Part model, mm, in its own coordinate system. Face numbers are marked on the shaded views. A direction names the side the tool comes from. Round coordinates to 2 decimals unless told otherwise and drop trailing zeros. Write each loop counter-clockwise with the first axis right and the second up, starting at its lowest first coordinate (ties: lowest second). Pieces come first, ordered by that corner, then holes. Notation, with made-up numbers: M 86.5,-4.75 L 118.5,-4.75 A17 cw 118.5,4.25 Z; hole C 85.5,57.25 d4. An arc over 180 degrees is marked long. Use one line per item in the form item = value. Start each with the question number.
Item 1: Cut at A-A, the plane x = 15.5. Give the cut face in (y, z), then the cut area to 3 significant figures.
Item 2: Cut at D-D, the plane z = -15.5. Give the cut face in (x, y), then the cut area to 3 significant figures.
Item 3: Probe L1, parallel to X at y = 17, z = 31; L2, parallel to X at y = 1, z = -15; L3, parallel to Z at x = -15, y = 1. List the from-to ranges inside material, lowest first.
Item 4: Cut at B-B, the plane z = 0.5. Give the cut face in (x, y).
Item 5: Cut at C-C, the plane y = 17. Give the cut face in (x, z).
Item 6: Mould opens along X. For the marked faces 1, 2 and 3 say: +X half, -X half, draft (parallel to the pull), parting line (faces both ways), or undercut.
Item 7: Flat gauge pins, fed straight in: pin 1 Ø3.5 at (x, z) = (15.5, 15.5) entering from +Y; pin 2 Ø2 at (y, z) = (1, -3) entering from +X; pin 3 Ø1.8 at (x, z) = (-15.5, 15.5) entering from +Y; pin 4 Ø13 at (x, y) = (-24.68, 17) entering from -Z. Where does each tip first touch, or does it go through?
Item 8: Which spindle directions (+Z, -Z, +X, -X, +Y, -Y) get a long thin tool onto all of the face, cutting with end or side? Do the marked faces 4 and 5. Say none if no direction does.
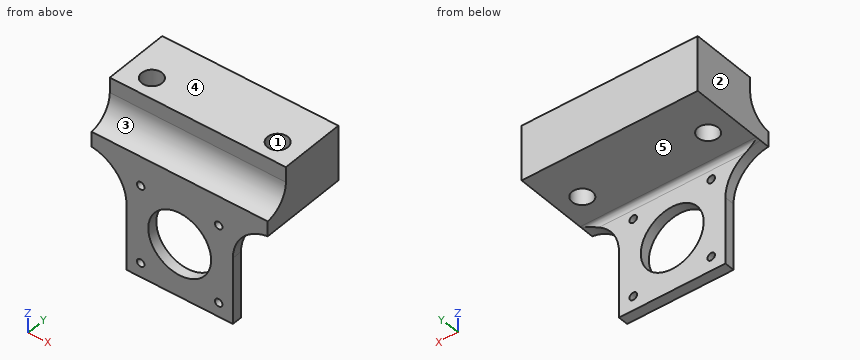
from build123d import *

# Parameters (mm, degrees)
SKETCH1_W           = 42.3
SKETCH1_H           = 42.3
SKETCH1_R           = 1.5
SKETCH1_R_2         = 12.5
BOSS_EXTRUDE1_DEPTH = 4
SKETCH2_W           = 70
SKETCH2_H           = 35
BOSS_EXTRUDE3_DEPTH = 6
SKETCH5_W           = 70
SKETCH5_H           = 26
SKETCH5_R           = 4.05
BOSS_EXTRUDE7_DEPTH = 16
CUT_EXTRUDE1_START  = -16
SKETCH5_2_R         = 4.05
CUT_EXTRUDE1_DEPTH  = 16
FILLET1_R           = 16
FILLET2_R           = 10
FILLET4_R           = 2


with BuildPart() as part:
    # Sketch1 → Boss-Extrude1 (new body)
    with BuildSketch(Plane(origin=(0, 0, 0), x_dir=(1, 0, 0), z_dir=(0, 1, 0))):
        Rectangle(SKETCH1_W, SKETCH1_H)
        with Locations(Location((-15.5, 15.5, 0), (0, 0, 270))):
            Circle(SKETCH1_R, mode=Mode.SUBTRACT)
        with Locations(Location((15.5, 15.5, 0), (0, 0, 270))):
            Circle(SKETCH1_R, mode=Mode.SUBTRACT)
        with Locations(Location((15.5, -15.5, 0), (0, 0, 270))):
            Circle(SKETCH1_R, mode=Mode.SUBTRACT)
        with Locations(Location((-15.5, -15.5, 0), (0, 0, 270))):
            Circle(SKETCH1_R, mode=Mode.SUBTRACT)
        with Locations(Location((0, 0, 0), (0, 0, 270))):
            Circle(SKETCH1_R_2, mode=Mode.SUBTRACT)
    extrude(amount=BOSS_EXTRUDE1_DEPTH)

    # Sketch2 → Boss-Extrude3 (add)
    with BuildSketch(Plane.XY.offset(21.15)):
        with Locations((0, 17.5)):
            Rectangle(SKETCH2_W, SKETCH2_H)
    extrude(amount=BOSS_EXTRUDE3_DEPTH)

    # Sketch5 → Boss-Extrude7 (add)
    with BuildSketch(Plane.XY.offset(27.15)):
        with Locations((0, 22)):
            Rectangle(SKETCH5_W, SKETCH5_H)
        with Locations((-24.679036529, 17)):
            Circle(SKETCH5_R, mode=Mode.SUBTRACT)
        with Locations((25.320963471, 17)):
            Circle(SKETCH5_R, mode=Mode.SUBTRACT)
    extrude(amount=BOSS_EXTRUDE7_DEPTH)

    # Sketch5<2> → Cut-Extrude1 (cut)
    with BuildSketch(Plane.XY.offset(27.15).offset(CUT_EXTRUDE1_START)):
        with Locations((-24.679036529, 17)):
            Circle(SKETCH5_2_R)
        with Locations((25.320963471, 17)):
            Circle(SKETCH5_2_R)
    extrude(amount=CUT_EXTRUDE1_DEPTH, mode=Mode.SUBTRACT)

    # Fillet1
    # the kernel refuses this fillet: 16 mm, written as the material it adds along each edge
    with BuildSketch(Plane(origin=(21.15, 0, 21.15), x_dir=(1, 0, 0), z_dir=(0, 1, 0))) as fillet1_piece_1:
        with BuildLine():
            CenterArc((16, 15.854888836), FILLET1_R, 180, 82.27751927)
            Line((0, 15.854888836), (-0.32, 15.854888836))
            Line((-0.32, 15.854888836), (-0.32, 0))
            Line((-0.32, 0), (0, -0.32))
            ThreePointArc((0, -0.32), (6.925, -0.32), (13.807, -0.317097777))
            Line((13.807, -0.317097777), (13.85, 0))
        make_face()
    extrude(amount=4)
    with BuildSketch(Plane(origin=(-21.15, 0, 21.15), x_dir=(-1, 0, 0), z_dir=(0, 1, 0))) as fillet1_piece_2:
        with BuildLine():
            CenterArc((16, -15.854888836), FILLET1_R, 97.72248073, 82.27751927)
            Line((0, -15.854888836), (-0.32, -15.854888836))
            Line((-0.32, -15.854888836), (-0.32, 0))
            Line((-0.32, 0), (0, 0.32))
            ThreePointArc((0, 0.32), (6.925, 0.32), (13.807, 0.317097777))
            Line((13.807, 0.317097777), (13.85, 0))
        make_face()
    extrude(amount=4)

    # Fillet2
    # the kernel refuses this fillet: 10 mm, written as the material it adds along each edge
    with BuildSketch(Plane(origin=(35, 9, 27.15), x_dir=(0, 0, 1), z_dir=(-1, 0, 0))) as fillet2_piece_1:
        with BuildLine():
            CenterArc((9.949874371, -10), FILLET2_R, 90, 84.260829523)
            Line((0, -9), (-0.198997487, -8.98))
            ThreePointArc((-0.198997487, -8.98), (-0.2, -4.5), (-0.2, 0))
            Line((-0.2, 0), (0, 0.2))
            Line((0, 0.2), (9.949874371, 0.2))
            Line((9.949874371, 0.2), (9.949874371, 0))
        make_face()
    extrude(amount=70)

    # Fillet4
    # the kernel refuses this fillet: 2 mm, written as the material it adds along each edge
    with BuildSketch(Plane(origin=(-35, 4, 21.15), x_dir=(0, 1, 0), z_dir=(1, 0, 0))) as fillet4_piece_1_section:
        with BuildLine():
            CenterArc((FILLET4_R, -FILLET4_R), FILLET4_R, 90, 90)
            Line((0, -FILLET4_R), (0, 0))
            Line((0, 0), (FILLET4_R, 0))
        make_face()
    fillet4_piece_1 = extrude(amount=70, mode=Mode.PRIVATE)
    fillet4_piece_1 = fillet4_piece_1 - Plane(origin=(-37.15, 4.464640399, 5.295111164), x_dir=(-1, 0, 0), z_dir=(0, -1, 0)) * Cylinder(16, 148, mode=Mode.PRIVATE)
    fillet4_piece_1 = fillet4_piece_1 - Plane(origin=(37.15, 4.464640399, 5.295111164), x_dir=(1, 0, 0), z_dir=(0, -1, 0)) * Cylinder(16, 148, mode=Mode.PRIVATE)
    add(fillet4_piece_1)


solid = part.part
Model answer:
q1.outline = M 0,-21.15 L 4,-21.15 L 4,-17 L 0,-17 Z; M 0,-14 L 4,-14 L 4,14 L 0,14 Z; M 0,17 L 4,17 L 4,19.15 A2 cw 6,21.15 L 35,21.15 L 35,43.15 L 9,43.15 L 9,37.1 A10 cw 0,27.15 Z
q1.area = 793 mm²
q2.outline = M -21.15,0 L -17,0 L -17,4 L -21.15,4 Z; M -14,0 L 14,0 L 14,4 L -14,4 Z; M 17,0 L 21.15,0 L 21.15,4 L 17,4 Z
q2.area = 145 mm²
q3.L1 = -35 to -28.73, -20.63 to 21.27, 29.37 to 35
q3.L2 = -21.15 to -16.91, -14.09 to 14.09, 16.91 to 21.15
q3.L3 = -21.15 to -16.91, -14.09 to 14.09, 16.91 to 27.3
q4.outline = M -21.15,0 L -12.49,0 L -12.49,4 L -21.15,4 Z; M 12.49,0 L 21.15,0 L 21.15,4 L 12.49,4 Z
q5.outline = M -35,21.15 L -28.73,21.15 L -28.73,43.15 L -35,43.15 Z; M -20.63,21.15 L 21.27,21.15 L 21.27,43.15 L -20.63,43.15 Z; M 29.37,21.15 L 35,21.15 L 35,43.15 L 29.37,43.15 Z
q6.face_1 = undercut
q6.face_2 = -X half
q6.face_3 = draft
q7.pin_1 = 4
q7.pin_2 = 21.15
q7.pin_3 = through
q7.pin_4 = 21.15
q8.face_4 = +Z, +X, -X, +Y, -Y
q8.face_5 = -Z, +X, -X, +Y
